```python
from build123d import *

# Parameters (mm, degrees)
ESQUISSE1_W                  = 102
ESQUISSE1_H                  = 100
BOSS_EXTRU_1_DEPTH           = 4
ESQUISSE2_W                  = 5
ESQUISSE2_H                  = 100
BOSS_EXTRU_2_DEPTH           = 35
ENL_V_MAT_EXTRU_1_DEPTH      = 149.07092895
ENL_V_MAT_EXTRU_1_DEPTH_BACK = 149.07092895
ESQUISSE3_R                  = 3.5
ENL_V_MAT_EXTRU_2_DEPTH      = 149.07092895
ENL_V_MAT_EXTRU_2_DEPTH_BACK = 149.07092895
CONG_1_R                     = 10
ENL_V_MAT_EXTRU_3_DEPTH      = 148.068011478
ENL_V_MAT_EXTRU_3_DEPTH_BACK = 148.068011478
ESQUISSE5_W                  = 37
ESQUISSE5_H                  = 41
CONG_2_R                     = 3
CHANFREIN1_SIZE              = 2


with BuildPart() as part:
    # Esquisse1 → Boss.-Extru.1 (new body)
    with BuildSketch(Plane.XY):
        with Locations((51, 50)):
            Rectangle(ESQUISSE1_W, ESQUISSE1_H)
    extrude(amount=BOSS_EXTRU_1_DEPTH)

    # Esquisse2 → Boss.-Extru.2 (add)
    with BuildSketch(Plane.XY.offset(4)):
        with Locations((2.5, 50)):
            Rectangle(ESQUISSE2_W, ESQUISSE2_H)
        with Locations((99.5, 50)):
            Rectangle(ESQUISSE2_W, ESQUISSE2_H)
    extrude(amount=BOSS_EXTRU_2_DEPTH)

    # Esquisse3 → Enlèv. mat.-Extru.1 (cut, two sides: drawn at the far end of the back side and taken through both)
    with BuildSketch(Plane.ZY.offset(-ENL_V_MAT_EXTRU_1_DEPTH_BACK)):
        with Locations(Location((22, 12, 0), (0, 0, 270))):
            Circle(ESQUISSE3_R)
        with Locations(Location((22, 88, 0), (0, 0, 270))):
            Circle(ESQUISSE3_R)
    extrude(amount=ENL_V_MAT_EXTRU_1_DEPTH + ENL_V_MAT_EXTRU_1_DEPTH_BACK, mode=Mode.SUBTRACT)

    # Esquisse4 → Enlèv. mat.-Extru.2 (cut, two sides: drawn at the far end of the back side and taken through both)
    with BuildSketch(Plane.ZY.offset(-ENL_V_MAT_EXTRU_2_DEPTH_BACK)):
        Polygon((39, 82), (8, 66), (8, 34), (39, 18), align=None)
    extrude(amount=ENL_V_MAT_EXTRU_2_DEPTH + ENL_V_MAT_EXTRU_2_DEPTH_BACK, mode=Mode.SUBTRACT)

    # Congé1
    cong_1_edges = [part.edges().sort_by_distance(p)[0] for p in [
        (99.5, 100, 39),
        (99.5, 0, 39),
        (2.5, 0, 39),
        (2.5, 100, 39),
        (2.5, 82, 39),
        (2.5, 18, 39),
        (99.5, 82, 39),
        (2.5, 34, 8),
        (99.5, 34, 8),
        (99.5, 18, 39),
        (2.5, 66, 8),
        (99.5, 66, 8),
    ]]
    fillet(cong_1_edges, radius=CONG_1_R)

    # Esquisse5 → Enlèv. mat.-Extru.3 (cut, two sides: drawn at the far end of the back side and taken through both)
    with BuildSketch(Plane.XY.offset(4).offset(-ENL_V_MAT_EXTRU_3_DEPTH_BACK)):
        with Locations((29.5, 73.5)):
            Rectangle(ESQUISSE5_W, ESQUISSE5_H)
        with Locations((29.5, 26.5)):
            Rectangle(ESQUISSE5_W, ESQUISSE5_H)
        with Locations((72.5, 26.5)):
            Rectangle(ESQUISSE5_W, ESQUISSE5_H)
        with Locations((72.5, 73.5)):
            Rectangle(ESQUISSE5_W, ESQUISSE5_H)
    extrude(amount=ENL_V_MAT_EXTRU_3_DEPTH + ENL_V_MAT_EXTRU_3_DEPTH_BACK, mode=Mode.SUBTRACT)

    # Congé2
    cong_2_edges = [part.edges().sort_by_distance(p)[0] for p in [
        (54, 94, 2),
        (91, 94, 2),
        (91, 53, 2),
        (54, 53, 2),
        (91, 47, 2),
        (91, 6, 2),
        (54, 6, 2),
        (54, 47, 2),
        (48, 6, 2),
        (11, 6, 2),
        (11, 47, 2),
        (48, 47, 2),
        (11, 53, 2),
        (11, 94, 2),
        (48, 94, 2),
        (48, 53, 2),
    ]]
    fillet(cong_2_edges, radius=CONG_2_R)

    # Chanfrein1
    chanfrein1_edges = [part.edges().sort_by_distance(p)[0] for p in [
        (97, 50, 4),
        (5, 50, 4),
        (102, 50, 0),
        (0, 50, 0),
    ]]
    chamfer(chanfrein1_edges, length=CHANFREIN1_SIZE)


solid = part.part
```
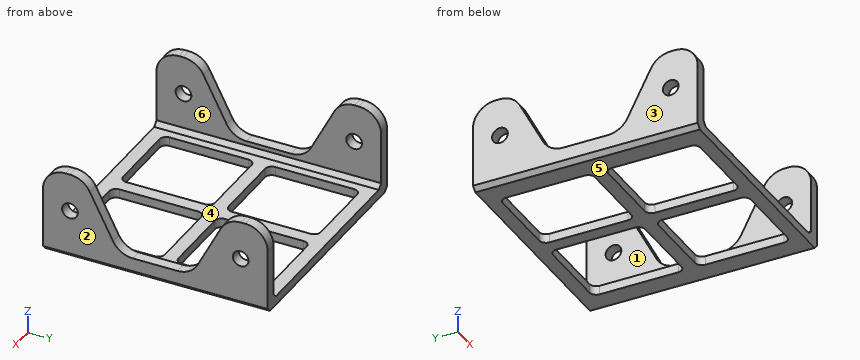
Work out the finished part from the listing and answer in its coordinate system (mm). Face numbers are marked on the shaded views. A direction names the side the tool comes from. Coordinates: 2 decimals unless noted, no trailing zeros. Loops run counter-clockwise (first coordinate to the right, second up) from the corner with the lowest first, then second, coordinate; pieces in that order, holes last. Notation, with made-up numbers: (77, -29.75) - (134, -29.75) arc R28 cw to (134, -7.75) - close; hole circle Ø11 at (79.5, 27). An arc over 180 degrees is marked (long way). Use a Markdown table: item, result.
Item 1: Consider probe 1 along Z at (x, y) = (98.5, 12); probe 2 along Y at (x, z) = (98.1, 22); probe 3 along Y at (x, z) = (60.5, 3). Determine where each line is inside the solid, lowest interval first. Write a range as from..to.
Evaluation:
| item | result |
|---|---|
| probe 1 | z = 0..18.5, 25.5..39 |
| probe 2 | y = 0..8.5, 15.5..26.77, 73.23..84.5, 91.5..100 |
| probe 3 | y = 0..6, 47..53, 94..100 |
Item 2: The mould has two halves that part along X. Classify the marked faces 1, 2, 3 and 4: +X half, -X half, draft (parallel to the pull), parting line (faces both ways), or undercut.
Evaluation:
| item | result |
|---|---|
| face 1 | undercut |
| face 2 | +X half |
| face 3 | -X half |
| face 4 | undercut |
Item 3: Find section D-D, the plane z = 10.5. Determine the outline of the cut face in (x, y), and give its area (3 significant figures).
Evaluation:
| item | result |
|---|---|
| outline | (0, 0) - (5, 0) - (5, 33.48) - (0, 33.48) - close; (0, 66.52) - (5, 66.52) - (5, 100) - (0, 100) - close; (97, 0) - (102, 0) - (102, 33.48) - (97, 33.48) - close; (97, 66.52) - (102, 66.52) - (102, 100) - (97, 100) - close |
| area | 670 mm2 |
Item 4: For the marked faces 5 and 6, determine the directions among +Z, -Z, +X, -X, +Y, -Y from which every point of the face is accessible in a straight line to the end or side of a thin tool.
Evaluation:
| item | result |
|---|---|
| face 5 | -Z, +X, -X, +Y, -Y |
| face 6 | +Z, +Y, -Y |
Item 5: Given pin 1 Ø6 at (x, y) = (89, 65.5) entering from +Z; pin 2 Ø1.5 at (x, y) = (99, 50) entering from +Z, each flat-ended and moving along its own axis, determine where each tip first touches the part or whether it passes through.
Evaluation:
| item | result |
|---|---|
| pin 1 | stops at z = 4 |
| pin 2 | stops at z = 8 |
Item 6: Find section A-A, the plane x = 16. Determine the outline of the cut face in (y, z).
Evaluation:
| item | result |
|---|---|
| outline | (0, 0) - (6, 0) - (6, 4) - (0, 4) - close; (47, 0) - (53, 0) - (53, 4) - (47, 4) - close; (94, 0) - (100, 0) - (100, 4) - (94, 4) - close |
Item 7: Find section C-C, the plane y = 14. Determine the outline of the cut face in (x, z), and give its area (3 significant figures).
Evaluation:
| item | result |
|---|---|
| outline | (0, 2) - (2, 0) - (11, 0) - (11, 4) - (7, 4) - (5, 6) - (5, 19.13) - (0, 19.13) - close; (0, 24.87) - (5, 24.87) - (5, 38.78) - (0, 38.78) - close; (48, 0) - (54, 0) - (54, 4) - (48, 4) - close; (91, 0) - (100, 0) - (102, 2) - (102, 19.13) - (97, 19.13) - (97, 6) - (95, 4) - (91, 4) - close; (97, 24.87) - (102, 24.87) - (102, 38.78) - (97, 38.78) - close |
| area | 402 mm2 |
Item 8: Find section B-B, the plane z = 22. State how many separate pieces and enclosed holes the cut face has, and give its area (3 significant figures).
Evaluation:
| item | result |
|---|---|
| separate pieces | 8 |
| enclosed holes | 0 |
| area | 395 mm2 |
